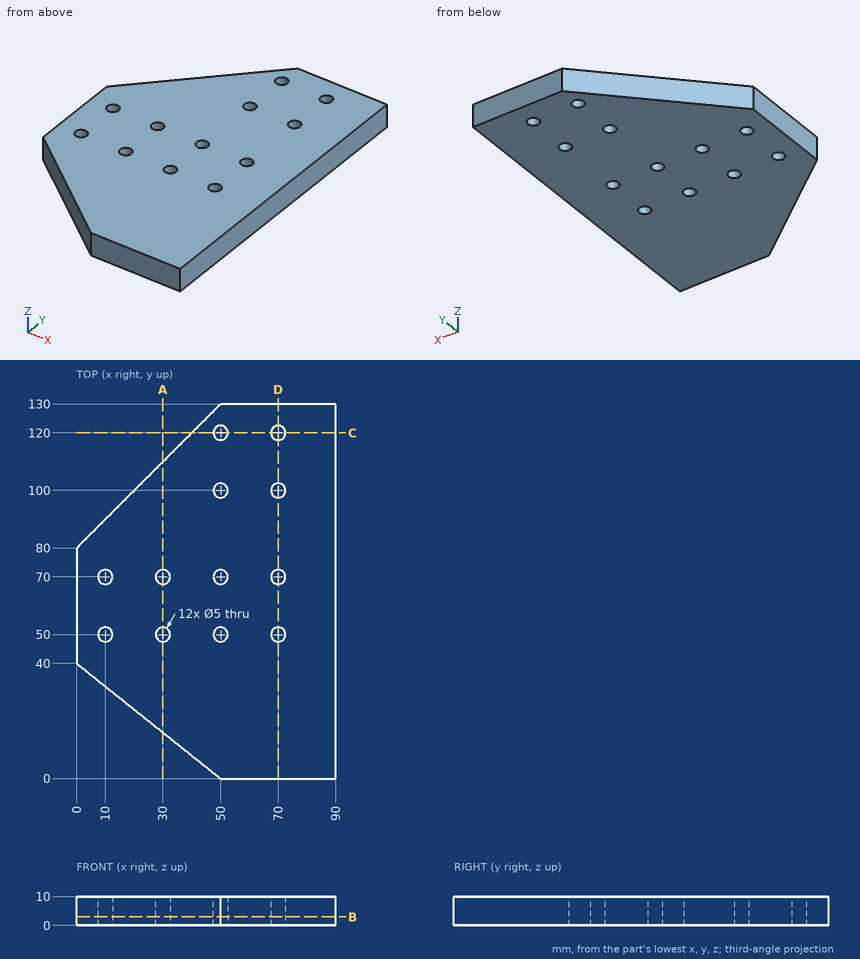
The figure shows three views and two pictorial views of one solid part (mm, origin at its lowest corner). Answer the questions. Coordinates: 2 decimals unless noted, no trailing zeros. Loops run counter-clockwise (first coordinate to the right, second up) from the corner with the lowest first, then second, coordinate; pieces in that order, holes last. Notation, with made-up numbers: (57.25, 71.5) -> (75.25, 71.5) arc R9 cw to (75.25, 88.5) -> close; hole circle Ø5 at (74.25, -32). An arc over 180 degrees is marked (long way). Return JSON: item names as keys, results as strings. Group by question number.
(1) Given pin 1 Ø2 at (x, z) = (46.5, 7.5) entering from -Y; pin 2 Ø4.5 at (x, y) = (50, 70) entering from -Z; pin 3 Ø5 at (y, z) = (102.5, 4.5) entering from -X; pin 4 Ø5 at (x, z) = (26.5, 8.5) entering from -Y, each flat-ended and moving along its own axis, determine where each tip first touches the part or whether it passes through.
(2) A cutting plane is placed at B-B on z = 3. Count the separate pieces of the cut face and the enclosed holes in it, and give its area (3 significant figures).
(3) A cutting plane is placed at A-A on x = 30. Write down the section's boundary in (y, z), and give its area (3 significant figures).
(4) A cutting plane is placed at C-C on y = 120. Write down the section's boundary in (x, z), and give its area (3 significant figures).
(5) A cutting plane is placed at D-D on x = 70. Write down the section's boundary in (y, z), and give its area (3 significant figures).
(6) Find the intervals of material crossed by probe 1 along Y at (x, z) = (48, 7.75); probe 2 along Y at (x, z) = (10, 8); probe 3 along Y at (x, z) = (30, 6.25), in increasing order. Write a range as from..to.
The answers:
{
 "1": {"pin 1": "stops at y = 2", "pin 2": "passes through", "pin 3": "stops at x = 20", "pin 4": "stops at y = 16.8"},
 "2": {"separate pieces": "1", "enclosed holes": "12", "area": "9,210 mm^2"},
 "3": {"outline": "(16, 0) -> (47.5, 0) -> (47.5, 10) -> (16, 10) -> close; (52.5, 0) -> (67.5, 0) -> (67.5, 10) -> (52.5, 10) -> close; (72.5, 0) -> (110, 0) -> (110, 10) -> (72.5, 10) -> close", "area": "840 mm^2"},
 "4": {"outline": "(40, 0) -> (47.5, 0) -> (47.5, 10) -> (40, 10) -> close; (52.5, 0) -> (67.5, 0) -> (67.5, 10) -> (52.5, 10) -> close; (72.5, 0) -> (90, 0) -> (90, 10) -> (72.5, 10) -> close", "area": "400 mm^2"},
 "5": {"outline": "(0, 0) -> (47.5, 0) -> (47.5, 10) -> (0, 10) -> close; (52.5, 0) -> (67.5, 0) -> (67.5, 10) -> (52.5, 10) -> close; (72.5, 0) -> (97.5, 0) -> (97.5, 10) -> (72.5, 10) -> close; (102.5, 0) -> (117.5, 0) -> (117.5, 10) -> (102.5, 10) -> close; (122.5, 0) -> (130, 0) -> (130, 10) -> (122.5, 10) -> close", "area": "1,100 mm^2"},
 "6": {"probe 1": "y = 1.6..48.5, 51.5..68.5, 71.5..98.5, 101.5..118.5, 121.5..128", "probe 2": "y = 32..47.5, 52.5..67.5, 72.5..90", "probe 3": "y = 16..47.5, 52.5..67.5, 72.5..110"}
}
